Autodesk Inventor part; units mm, degrees
ref_plane "YZ Plane" through (0, 0, 0) normal (1, 0, 0) x (0, 1, 0)
ref_plane "XZ Plane" through (0, 0, 0) normal (0, 1, 0) x (-1, 0, 0)
ref_plane "XY Plane" through (0, 0, 0) normal (0, 0, 1) x (1, 0, 0)
sketch "Sketch1" plane through (0, 0, 0) normal (0, 0, 1) x (1, 0, 0)
  circle A0 centre (0, 0) radius 11
  circle A1 centre (0, 84) radius 14
  circle A2 centre (0, 0) radius 72 construction
  circle A3 centre (0, 84) radius 12 construction
  line L0 (0, 84) -> (0, 0) construction
  line L1 (-67.6579, 24.6255) -> (0, 0) construction
  line L2 (67.6579, 24.6255) -> (0, 0) construction
  circle A4 centre (0, 84) radius 35 construction
  line L3 (-60, 71.9226) -> (-60, 144)
  line L4 (-60, 144) -> (60, 144)
  line L5 (60, 144) -> (60, 71.9226)
  circle A5 centre (0, 0) radius 27.5
  line L6 (25.3583, -10.6399) -> (60, 71.9226)
  line L7 (-60, 71.9226) -> (-25.3583, -10.6399)
  line L8 (0, 0) -> (135.9462, -63.3927) construction
  line L9 (-24.7487, 59.2513) -> (24.7487, 59.2513) construction
  circle A6 centre (0, 84) radius 60
  point P0 (24.7487, 108.7487)
  point P1 (-24.7487, 108.7487)
  point P2 (55.3272, 60.7857)
  point P3 (-55.3272, 60.7857)
  dimension "d7" = 70
  dimension "d1" = 24
  dimension "d2" = 144
  dimension "d3" = 28
  dimension "d4" = 22
  dimension "d6" = 220
  dimension "d10" = 360
  dimension "d12" = 55
  dimension "d17" = 150
  dimension "d18" = 45
  dimension "d28" = 120
sketch "Sketch2" plane through (0, 0, 0) normal (0, 0, 1) x (1, 0, 0)
  point P0 (0, 0)
extrude "Extrusion1" add sketch "Sketch1" against normal blind 6 contours A6 A5 | A6 A5 L7 | A5 A6 | A5 A6 | A5 A6 L6
hole "Hole1" at (-24.7487, 59.2513, 0) at (-24.7487, 108.7487, 0) at (24.7487, 108.7487, 0) at (24.7487, 59.2513, 0) direction (0, 0, -1) diameter 5.8 end through all counterbore diameter 10 counterbore depth 5
sketch "Sketch3" plane through (0, 0, -6) normal (0, 0, -1) x (-1, 0, 0)
  circle A0 centre (0, 84) radius 50 construction
  line L0 (0, 84) -> (0, 134) construction
  circle A1 centre (0, 84) radius 14 construction
  line L1 (-49.2404, 75.3176) -> (0, 84) construction
  point P0 (0, 0)
  point P1 (-27.4754, 125.7744)
  point P2 (27.4754, 125.7744)
  point P3 (49.2404, 75.3176)
  dimension "d29" = 100
  dimension "d30" = 100
  dimension "d33" = 200
hole "Hole2" at (0, 84, -6) at (49.2404, 75.3176, -6) at (27.4754, 125.7744, -6) at (-27.4754, 125.7744, -6) at (-49.2404, 75.3176, -6) direction (0, 0, 1) diameter 4.8 end through all counterbore diameter 8 counterbore depth 4
equation "\"d2\" = 6 * d1"
properties part number "RT_ARM_MC_008_Capstand_Base"
Can you work these out from the model? Positions are in its coordinate system, mm. A direction names the side the tool comes from. Give positions to 0.01 mm unless a question says otherwise; leave off trailing zeros. Order: outer loops, then holes, each group sorted by start corner. A loop starts at its lowest first (then second) coordinate and runs counter-clockwise, first axis right, second up. Notation, with made-up numbers: M 41.25,-7 L 87.25,-7 A9 cw 87.25,5 Z; hole C -32,17 d11. An arc over 180 degrees is marked long. One line per question, with ' | ' between items.
Item 1: I'm going to push flat-ended pins straight in: pin 1 Ø16 at (x, y) = (24.75, 59.25) entering from +Z; pin 2 Ø9.5 at (x, y) = (-24.75, 108.75) entering from +Z; pin 3 Ø4.5 at (x, y) = (-49.24, 75.32) entering from +Z; pin 4 Ø1 at (x, z) = (-0.5, -1.5) entering from -Y. Where does each tip first touch, or does it pass through?
Answer block:
pin 1: stops at z = 0 | pin 2: stops at z = -5 | pin 3: passes through | pin 4: stops at y = -27.5
Item 2: Suppose I cut it at B-B, the plane y = 84. Write out the boundary of the cut face in (x, z).
Answer block:
outline: M -60,-6 L -14,-6 L -14,0 L -60,0 Z; M 14,-6 L 60,-6 L 60,0 L 14,0 Z
Item 3: For faces 5 (the face through (-1, 59, 0)), 6 (the face through (-25.94, 129.47, -3.97)), 7 (the face through (-25, 105, -5)), which set-ups out of +Z, -Z, +X, -X, +Y, -Y let a thin tool reach every point of the face, with its end or its side?
Answer block:
face 5: +Z, +X, -X, +Y, -Y | face 6: -Z | face 7: +Z
Item 4: We'd pull the mould along Y, two halves only. Please class faces 1 (the face through (1.653, 143.977, -2.958)), 2 (the face through (-24.876, 111.646, -5.507)), 3 (the face through (30.1, 125.7, -2)), 4 (the face through (-1, 59, -6)): released by +Y, released by -Y, zero draft, split by the parting line, or undercut.
Answer block:
face 1: split by the parting line | face 2: undercut | face 3: undercut | face 4: zero draft
Item 5: Please list where these lines run through material, in increasing order: L1, parallel to Y at x = -26.5, z = -3.45; L2, parallel to Y at x = -6.5, z = -5.55; L3, parallel to Y at x = -3.5, z = -0.4.
Answer block:
L1: y = -7.92 to 54.57, 63.93 to 104.07, 113.43 to 121.9, 129.65 to 137.83 | L2: y = -26.72 to -8.87, 8.87 to 71.6, 96.4 to 143.65 | L3: y = -27.28 to -10.43, 10.43 to 70.44, 97.56 to 143.9
Item 6: Suppose I cut it at D-D, the plane y = 0. Write out the boundary of the cut face in (x, z).
Answer block:
outline: M -29.82,-6 L -11,-6 L -11,0 L -29.82,0 Z; M 11,-6 L 29.82,-6 L 29.82,0 L 11,0 Z
Item 7: Suppose I cut it at A-A, the plane x = 0. Write out the boundary of the cut face in (y, z), then the cut area to 3 significant figures.
Answer block:
outline: M -27.5,-6 L -11,-6 L -11,0 L -27.5,0 Z; M 11,-6 L 70,-6 L 70,0 L 11,0 Z; M 98,-6 L 144,-6 L 144,0 L 98,0 Z | area: 729 mm2
Item 8: Suppose I cut it at C-C, the plane z = -2.9. Give the number of separate pieces and of enclosed holes in the cut face, then the cut area to 3 significant figures.
Answer block:
separate pieces: 1 | enclosed holes: 10 | area: 13,200 mm2
